Design review of the part built by this model. Coordinates are the model's own, in mm. Give positions to 0.01 mm unless a question says otherwise; leave off trailing zeros. Write each loop counter-clockwise with the first axis right and the second up, starting at its lowest first coordinate (ties: lowest second). Pieces come first, ordered by that corner, then holes.
```python
from build123d import *

# Parameters (mm, degrees)
SKETCH1_R           = 3.81
SKETCH1_R_2         = 3.429
BOSS_EXTRUDE1_DEPTH = 10.16


with BuildPart() as part:
    # Sketch1 → Boss-Extrude1 (new body)
    with BuildSketch(Plane.XY):
        Polygon((0, 0), (38.1, 0), (63.5, 127), (63.5, 190.5), (-25.4, 190.5), (-25.4, 125.291623319), align=None)
        with Locations((19.05, 12.7)):
            Circle(SKETCH1_R, mode=Mode.SUBTRACT)
        with Locations((19.05, 50.8)):
            Circle(SKETCH1_R, mode=Mode.SUBTRACT)
        with Locations((-6.35, 174.687730396)):
            Circle(SKETCH1_R_2, mode=Mode.SUBTRACT)
        with Locations((-6.35, 149.287730396)):
            Circle(SKETCH1_R_2, mode=Mode.SUBTRACT)
        with Locations(Location((44.45, 149.287730396, 0), (0, 0, 180))):
            Circle(SKETCH1_R_2, mode=Mode.SUBTRACT)
        with Locations(Location((44.45, 174.687730396, 0), (0, 0, 180))):
            Circle(SKETCH1_R_2, mode=Mode.SUBTRACT)
    extrude(amount=BOSS_EXTRUDE1_DEPTH)


solid = part.part
```
(1) Mouldability with a two-part tool opening along Y and no side actions: class faces 1 (the face through (19, 0, 5)), 2 (the face through (-25.4, 158, 5)), 3 (the face through (-6.796, 152.688, 5.009)) as pulls with the +Y half, pulls with the -Y half, needs draft (parallel to the pull), parting line crosses it, or undercut.
Resolved:
face 1: pulls with the -Y half
face 2: needs draft
face 3: undercut
(2) Consider section D-D, the plane x = -6.35. Give the boundary of the cut face in (y, z), then the cut area to 3 significant figures.
Resolved:
outline: (31.32, 0) - (145.86, 0) - (145.86, 10.16) - (31.32, 10.16) - close; (152.72, 0) - (171.26, 0) - (171.26, 10.16) - (152.72, 10.16) - close; (178.12, 0) - (190.5, 0) - (190.5, 10.16) - (178.12, 10.16) - close
area: 1,480 mm2
(3) Consider section A-A, the plane x = 19.05. Give the boundary of the cut face in (y, z), then the cut area to 3 significant figures.
Resolved:
outline: (0, 0) - (8.89, 0) - (8.89, 10.16) - (0, 10.16) - close; (16.51, 0) - (46.99, 0) - (46.99, 10.16) - (16.51, 10.16) - close; (54.61, 0) - (190.5, 0) - (190.5, 10.16) - (54.61, 10.16) - close
area: 1,780 mm2
(4) Consider section C-C, the plane y = 12.7. Give the boundary of the cut face in (x, z).
Resolved:
outline: (-2.57, 0) - (15.24, 0) - (15.24, 10.16) - (-2.57, 10.16) - close; (22.86, 0) - (40.64, 0) - (40.64, 10.16) - (22.86, 10.16) - close
(5) To check wall thickness, follow L1, parallel to Y at x = 19.05, z = 5; L2, parallel to X at y = 96, z = 7.5; L3, parallel to X at y = 68, z = 4. State the ranges of each line that lie inside material, in increasing order.
Resolved:
L1: y = 0 to 8.89, 16.51 to 46.99, 54.61 to 190.5
L2: x = -19.46 to 57.3
L3: x = -13.79 to 51.7
(6) Clearance check with a flat-ended pin moving along its axis: P1, Ø4, axis at x = -6.35, y = 174.69, coming from the +Z side. State where the tip first meets the part, or that it passes through.
Resolved:
P1: passes through
(7) Consider section B-B, the plane z = 6.5. Give the boundary of the cut face in (x, y), then the cut area to 3 significant figures.
Resolved:
outline: (-25.4, 125.29) - (0, 0) - (38.1, 0) - (63.5, 127) - (63.5, 190.5) - (-25.4, 190.5) - close; hole circle Ø6.86 at (-6.35, 149.29); hole circle Ø6.86 at (-6.35, 174.69); hole circle Ø7.62 at (19.05, 12.7); hole circle Ø7.62 at (19.05, 50.8); hole circle Ø6.86 at (44.45, 149.29); hole circle Ø6.86 at (44.45, 174.69)
area: 13,500 mm2
